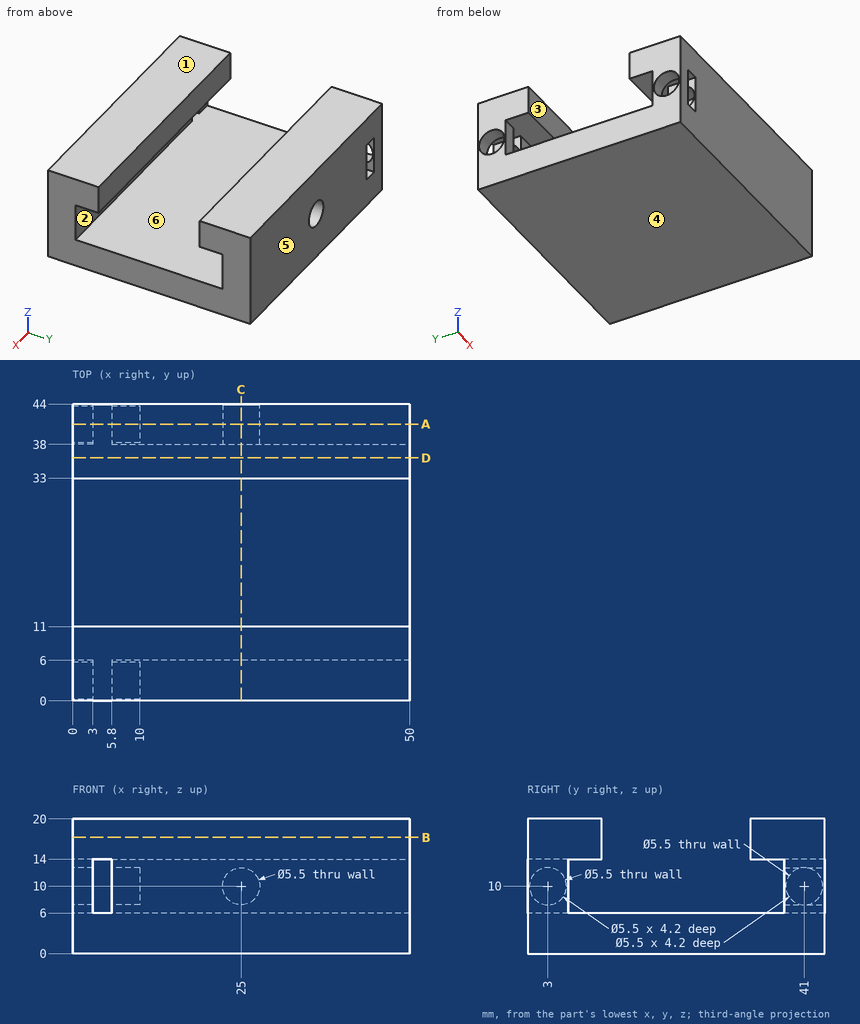
The figure shows three views and two pictorial views of one solid part (mm, origin at its lowest corner). Answer the questions. A direction names the side the tool comes from. Coordinates: 2 decimals unless noted, no trailing zeros. Order: outer loops, then holes, each group sorted by start corner. A loop starts at its lowest first (then second) coordinate and runs counter-clockwise, first axis right, second up. Notation, with made-up numbers: M 0.5,-35.5 L 19.5,-35.5 A27 cw 19.5,-11.5 Z; hole C 23,-22.75 d2. An arc over 180 degrees is marked long. Use CSV: the item, a comma, the result in double quotes.
1) Section A-A on y = 41 is taken. Write down the section's boundary in (x, z), plus the area to 3 significant figures.
Worked out:
outline,"M 0,0 L 50,0 L 50,20 L 0,20 L 0,12.75 L 3,12.75 L 3,14 L 5.8,14 L 5.8,12.75 L 10,12.75 L 10,7.25 L 5.8,7.25 L 5.8,6 L 3,6 L 3,7.25 L 0,7.25 Z; hole C 25,10 d5.5"
area,"914 mm^2"
2) Section B-B on z = 17.25 is taken. Write down the section's boundary in (x, y).
Worked out:
outline,"M 0,0 L 50,0 L 50,11 L 0,11 Z; M 0,33 L 50,33 L 50,44 L 0,44 Z"
3) Section D-D on y = 36 is taken. Write down the section's boundary in (x, z), plus the area to 3 significant figures.
Worked out:
outline,"M 0,0 L 50,0 L 50,6 L 0,6 Z; M 0,14 L 50,14 L 50,20 L 0,20 Z"
area,"600 mm^2"
4) Consider line 1 (Y direction, x = 7.5, z = 10); line 2 (Z direction, x = 1, y = 41); line 3 (Y direction, x = 21.5, z = 13.25). Determine where each line is inside the solid, lowest interval first. Write a range as [from, to].
Worked out:
line 1,"y = [0, 0.25], [5.75, 6], [38, 38.25], [43.75, 44]"
line 2,"z = [0, 7.25], [12.75, 20]"
line 3,"y = [0, 6], [38, 44]"
5) For the marked faces 1, 2 and 3, determine the directions among +Z, -Z, +X, -X, +Y, -Y from which every point of the face is accessible in a straight line to the end or side of a thin tool.
Worked out:
face 1,"+Z, +X, -X, +Y, -Y"
face 2,"+X, -X"
face 3,"+Z, +X, -X"
6) Section C-C on x = 25 is taken. Write down the section's boundary in (y, z), plus the area to 3 significant figures.
Worked out:
outline,"M 0,0 L 44,0 L 44,7.25 L 38,7.25 L 38,6 L 6,6 L 6,14 L 11,14 L 11,20 L 0,20 Z; M 33,14 L 38,14 L 38,12.75 L 44,12.75 L 44,20 L 33,20 Z"
area,"459 mm^2"
7) Flat-ended cylindrical pins translate along their axes: pin 1 Ø1.8 at (y, z) = (3.5, 11) entering from -X; pin 2 Ø5 at (x, y) = (40, 28) entering from +Z. Find the tip coordinate at first contact, or state that the pin passes through.
Worked out:
pin 1,"stops at x = 10"
pin 2,"stops at z = 6"
8) Determine the mould class of the marked faces 4, 5 and 6 for opening direction Z: released by +Z, released by -Z, zero draft, split by the parting line, or undercut.
Worked out:
face 4,"released by -Z"
face 5,"zero draft"
face 6,"undercut"
